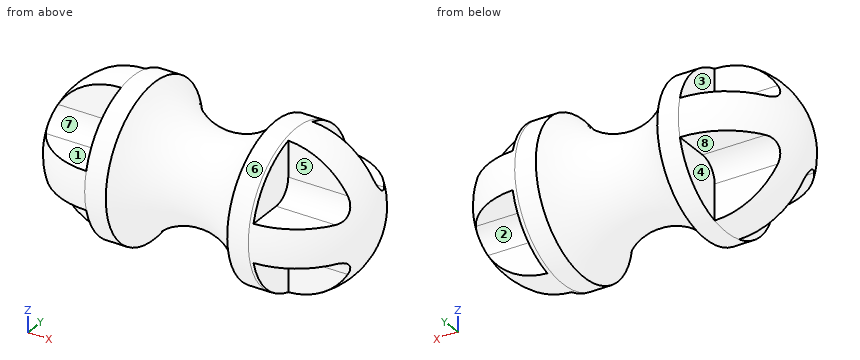
```python
from build123d import *

# Parameters (mm, degrees)
CUT_EXTRUDE1_DEPTH = 110


with BuildPart() as part:
    # Sketch1 → Revolve1 (revolve)
    with BuildSketch(Plane(origin=(0, 0, 0), x_dir=(1, 0, 0), z_dir=(0, 1, 0)), mode=Mode.PRIVATE) as revolve1_sk:
        with BuildLine():
            Line((-43.842141265, 39.917998991), (-32.781970874, 39.917998991))
            ThreePointArc((-32.781970874, 39.917998991), (-0.947206756, 22.460391682), (30.887557363, 39.917998991))
            Line((30.887557363, 39.917998991), (41.947727754, 39.917998991))
            ThreePointArc((41.947727754, 39.917998991), (70.174015532, 28.226287778), (81.865726745, 0))
            Line((81.865726745, 0), (-83.760140257, 0))
            ThreePointArc((-83.760140257, 0), (-72.068429044, 28.226287778), (-43.842141265, 39.917998991))
        make_face()
    revolve(revolve1_sk.sketch.rotate(Axis((-43.842141265, 0, 0), (1, 0, 0)), 180), axis=Axis((-43.842141265, 0, 0), (1, 0, 0)))

    # Sketch2 → Cut-Extrude1 (cut)
    with BuildSketch(Plane(origin=(-43.842141265, 0, 0), x_dir=(0, 0, -1), z_dir=(1, 0, 0))):
        with BuildLine():
            Line((-10, 38.645137385), (-10, 20))
            ThreePointArc((-10, 20), (-12.928932188, 12.928932188), (-20, 10))
            Line((-20, 10), (-38.645137385, 10))
            ThreePointArc((-38.645137385, 10), (-28.226287778, 28.226287778), (-10, 38.645137385))
        make_face()
        with BuildLine():
            Line((10, 38.645137385), (10, 20))
            ThreePointArc((10, 20), (12.928932188, 12.928932188), (20, 10))
            Line((20, 10), (38.645137385, 10))
            ThreePointArc((38.645137385, 10), (28.226287778, 28.226287778), (10, 38.645137385))
        make_face()
        with BuildLine():
            Line((-38.645137385, -10), (-20, -10))
            ThreePointArc((-20, -10), (-12.928932188, -12.928932188), (-10, -20))
            Line((-10, -20), (-10, -38.645137385))
            ThreePointArc((-10, -38.645137385), (-28.226287778, -28.226287778), (-38.645137385, -10))
        make_face()
        with BuildLine():
            Line((10, -20), (10, -38.645137385))
            ThreePointArc((10, -38.645137385), (28.226287778, -28.226287778), (38.645137385, -10))
            Line((38.645137385, -10), (20, -10))
            ThreePointArc((20, -10), (12.928932188, -12.928932188), (10, -20))
        make_face()
    cut_extrude1 = extrude(amount=-CUT_EXTRUDE1_DEPTH, mode=Mode.SUBTRACT)

    # Mirror1: Cut-Extrude1 across plane
    add(cut_extrude1.mirror(Plane(origin=(0, 0, 0), x_dir=(0, 0, 1), z_dir=(1, 0, 0))), mode=Mode.SUBTRACT)


solid = part.part
```
CAD build for the part. Positions are in the model's coordinates, mm. Face numbers are marked on the shaded views. A direction names the side the tool comes from. Round coordinates to 2 decimals unless told otherwise and drop trailing zeros. Loops run counter-clockwise (first coordinate to the right, second up) from the corner with the lowest first, then second, coordinate; pieces in that order, holes last. Notation, with made-up numbers: M -11,25.5 L 37,25.5 A31 ccw 37,55.5 Z; hole C 1,86 d3. An arc over 180 degrees is marked long. Use a Markdown table: item, result. Add a question column.
(1) Flat gauge pins, fed straight in: pin 1 (20.5 mm diameter, centred on x = -60, y = -32.5, fed in from -Z); pin 2 (8 mm diameter, centred on x = -4, y = 4.5, fed in from -Z); pin 3 (20.5 mm diameter, centred on x = -67.5, z = -32.5, fed in from -Y). Where does each tip first touch, or does it go through?
(2) Cut at A-A (y = 0). Give the cut face in (x, z), and give its area (3 significant figures).
(3) Drill centre lines: line 1 (X direction, y = -28, z = -4); line 2 (X direction, y = -35, z = 7.5); line 3 (Z direction, x = -70, y = 26). Where is each one in solid material? Low to high.
(4) Cut at D-D (x = 35.5). Give the cut face in (y, z).
(5) Which spindle directions (+Z, -Z, +X, -X, +Y, -Y) get a long thin tool onto all of the face, cutting with end or side? Do the marked faces 1, 2, 3, 4 and 5. Say none if no direction does.
(6) Cut at C-C (x = 68). Give the cut face in (y, z), and give its area (3 significant figures).
(7) Pull direction Y, two halves, no side cores. Call the marked faces 6, 7 and 8: +Y half, -Y half, draft (parallel to the pull), parting line (faces both ways), or undercut.
Geometry says:
| question | item | result |
|---|---|---|
| 1 | pin 1 | stops at z = -10 |
| 1 | pin 2 | stops at z = -22.89 |
| 1 | pin 3 | stops at y = -10 |
| 2 | outline | M -43.84,-39.92 L -32.78,-39.92 A37.75 cw 30.89,-39.92 L 41.95,-39.92 A39.92 ccw 41.95,39.92 L 30.89,39.92 A37.75 cw -32.78,39.92 L -43.84,39.92 A39.92 ccw Z |
| 2 | area | 10,300 mm² |
| 3 | line 1 | x = -72.01 to -21.09, 19.2 to 70.12 |
| 3 | line 2 | x = -61.51 to -29.74, 27.85 to 59.62 |
| 3 | line 3 | z = -10 to 10 |
| 4 | outline | C 0,0 d79.84 |
| 5 | face 1 | +Z, -X, -Y |
| 5 | face 2 | -Z, +X, +Y |
| 5 | face 3 | +Z, -X, +Y |
| 5 | face 4 | -Z, -X, +Y |
| 5 | face 5 | +Z, +X, -Y |
| 6 | outline | M -28.54,-10 L -20,-10 A10 cw -10,-20 L -10,-28.54 A30.24 ccw 10,-28.54 L 10,-20 A10 cw 20,-10 L 28.54,-10 A30.24 ccw 28.54,10 L 20,10 A10 cw 10,20 L 10,28.54 A30.24 ccw -10,28.54 L -10,20 A10 cw -20,10 L -28.54,10 A30.24 ccw Z |
| 6 | area | 2,060 mm² |
| 7 | face 6 | parting line |
| 7 | face 7 | -Y half |
| 7 | face 8 | draft |
